Build history of the part. All positions in model axes, mm. A direction names the side the tool comes from. Coordinates: 2 decimals unless noted, no trailing zeros. Loops run counter-clockwise (first coordinate to the right, second up) from the corner with the lowest first, then second, coordinate; pieces in that order, holes last.
Item 1: Drill centre lines: line 1 along Y through (x, z) = (-159, 31.5); line 2 along Z through (x, y) = (188.5, -25); line 3 along Z through (x, y) = (158, -7). Where is each one in solid material? Low to high.
Item 2: Cut at B-B (y = -34). List the corners of the cut face in (x, z).
Item 3: 3-axis set-ups, long thin cutter, end or side, ignore diameter. For faces 1 (the face through (-436, -14, 3)), 2 (the face through (6, -4, 27)): which of +Z, -Z, +X, -X, +Y, -Y reach the whole face in a straight line?
Item 4: Flat gauge pins, fed straight in: pin 1 (6 mm diameter, centred on x = 73.5, z = 11.5, fed in from +Y); pin 2 (11.5 mm diameter, centred on x = -11.5, y = -18, fed in from +Z); pin 3 (1 mm diameter, centred on x = -128, z = 25.5, fed in from -Y); pin 4 (2 mm diameter, centred on y = -6, z = 25, fed in from -X). Where does each tip first touch, or does it go through?
Item 5: Cut at A-A (x = 267). List the corners of the cut face in (y, z).
Item 6: Cut at C-C (z = 25.5). List the corners of the cut face in (x, y), and give its area (3 significant figures).
from build123d import *

# Parameters (mm, degrees)
F1_DEPTH = 450
F3_DEPTH = 50.001


# Not quite as in the source:
# - a pattern or mirror of a feature is missing from the dataset's text; its kind, count and spacing are read off the source's solid


with BuildPart() as f1:
    # F0 (on Right) → F1 (new body, symmetric)
    with BuildSketch(Plane.YZ):
        with BuildLine():
            Line((0, 0), (0, 50))
            ThreePointArc((0, 50), (-2.8284271247, 48.8284271247), (-4, 46))
            Line((-4, 46), (-4, 8))
            ThreePointArc((-4, 8), (-5.1715728753, 5.1715728753), (-8, 4))
            Line((-8, 4), (-46, 4))
            ThreePointArc((-46, 4), (-48.8284271247, 2.8284271247), (-50, 0))
            Line((-50, 0), (0, 0))
        make_face()
    extrude(amount=F1_DEPTH, both=True)

    # F2 (on face) → F3 (cut, through all)
    with BuildSketch(Plane(origin=(0, 0, 0), x_dir=(1, 0, 0), z_dir=(0, 0, -1))):
        Polygon((400, 50), (450, 0), (450, 50), align=None)
    f3 = extrude(amount=-F3_DEPTH, mode=Mode.SUBTRACT)

    # F3_copies: F3 across plane
    add(f3.mirror(Plane(origin=(0, 0, 0), x_dir=(0, 0, -1), z_dir=(-1, 0, 0))), mode=Mode.SUBTRACT)


solid = f1.part
Filled sheet:
1. line 1: y = -4 to 0
1. line 2: z = 0 to 4
1. line 3: z = 0 to 4.13
2. outline: (-416, 0) - (416, 0) - (416, 4) - (-416, 4) - close
3. face 1: +Z, -Z, -X, -Y
3. face 2: +Z, +X, -X, -Y
4. pin 1: stops at y = 0
4. pin 2: stops at z = 4
4. pin 3: stops at y = -4
4. pin 4: passes through
5. outline: (-50, 0) - (0, 0) - (0, 50) arc R4 ccw to (-4, 46) - (-4, 8) arc R4 cw to (-8, 4) - (-46, 4) arc R4 ccw to start
6. outline: (-450, 0) - (-446, -4) - (446, -4) - (450, 0) - close
6. area: 3,580 mm2
